```python
from build123d import *

# Parameters (mm, degrees)
SKETCH1_W               = 8
SKETCH1_H               = 4.5
SKETCH1_R               = 1.5
SKETCH1_W_2             = 65.532
SKETCH1_H_2             = 78.229021166
SKETCH1_R_2             = 1.599939077
SKETCH1_R_3             = 1.6
SKETCH1_R_4             = 1.599995589
SKETCH1_W_3             = 59.532
SKETCH1_H_3             = 64.229021166
BOSS_EXTRUDE1_DEPTH     = 3
SKETCH2_W               = 40
SKETCH2_H               = 4
BOSS_EXTRUDE2_DEPTH     = 30
CUT_EXTRUDE1_DEPTH      = 111.01120349
CUT_EXTRUDE1_DEPTH_BACK = 111.01120349
SKETCH3_R               = 2
FILLET2_R               = 17
FILLET3_R               = 12
SKETCH1_8_W             = 65.532
SKETCH1_8_H             = 78.229021166
SKETCH1_8_R             = 1.599939077
SKETCH1_8_R_2           = 1.6
SKETCH1_8_R_3           = 1.599995589
SKETCH1_8_W_2           = 59.532
SKETCH1_8_H_2           = 64.229021166
BOSS_EXTRUDE3_DEPTH     = 20
SKETCH5_R               = 2.5
CUT_EXTRUDE2_DEPTH      = 5
SKETCH7_W               = 58.229021166
SKETCH7_H               = 14
CUT_EXTRUDE3_DEPTH      = 111.01120349


with BuildPart() as part:
    # Sketch1 → Boss-Extrude1 (new body)
    # profile 1 of 11: a face of its own
    with BuildSketch(Plane(origin=(0, 0, 0), x_dir=(1, 0, 0), z_dir=(0, 1, 0))):
        with Locations((-4, 59.114510583)):
            Rectangle(SKETCH1_W, SKETCH1_H)
        with Locations(Location((-4, 59.114510583, 0), (0, 0, 270))):
            Circle(SKETCH1_R, mode=Mode.SUBTRACT)
    # profile 2 of 11: a face of its own
    with BuildSketch(Plane(origin=(0, 0, 0), x_dir=(1, 0, 0), z_dir=(0, 1, 0))):
        with Locations((4, 59.114510583)):
            Rectangle(SKETCH1_W, SKETCH1_H)
    # profile 3 of 11: a face of its own
    with BuildSketch(Plane(origin=(0, 0, 0), x_dir=(1, 0, 0), z_dir=(0, 1, 0))):
        Polygon((0, 56.864510583), (0, 39.114510583), (32.766, 39.114510583), (28.9648375, 56.864510583), (20.483, 56.864510583), (20.483, 61.364510583), (28.0011625, 61.364510583), (24.2, 79.114510583), (0, 79.114510583), (0, 61.364510583), (8, 61.364510583), (8, 56.864510583), align=None)
    # profile 4 of 11: a face of its own
    with BuildSketch(Plane(origin=(0, 0, 0), x_dir=(1, 0, 0), z_dir=(0, 1, 0))):
        Polygon((20.483, 56.864510583), (28.9648375, 56.864510583), (28.0011625, 61.364510583), (20.483, 61.364510583), align=None)
    # profile 5 of 11: a face of its own
    with BuildSketch(Plane(origin=(0, 0, 0), x_dir=(1, 0, 0), z_dir=(0, 1, 0))):
        Polygon((28.0011625, 61.364510583), (28.9648375, 56.864510583), (36.483, 56.864510583), (36.483, 61.364510583), align=None)
        with Locations(Location((32.483, 59.114510583, 0), (0, 0, 270))):
            Circle(SKETCH1_R, mode=Mode.SUBTRACT)
    # profile 6 of 11: a face of its own
    with BuildSketch(Plane(origin=(0, 0, 0), x_dir=(1, 0, 0), z_dir=(0, 1, 0))):
        with Locations((32.766, 0)):
            Rectangle(SKETCH1_W_2, SKETCH1_H_2)
        with Locations(Location((39.450944, -35.179510583, 0), (0, 0, 270))):
            Circle(SKETCH1_R_2, mode=Mode.SUBTRACT)
        with Locations(Location((20.574, -35.179510583, 0), (0, 0, 270))):
            Circle(SKETCH1_R_3, mode=Mode.SUBTRACT)
        with Locations(Location((39.37, 35.1758104, 0), (0, 0, 270))):
            Circle(SKETCH1_R_2, mode=Mode.SUBTRACT)
        with Locations(Location((20.574, 35.1758104, 0), (0, 0, 270))):
            Circle(SKETCH1_R_4, mode=Mode.SUBTRACT)
        with Locations((32.766, 0)):
            Rectangle(SKETCH1_W_3, SKETCH1_H_3, mode=Mode.SUBTRACT)
    # profile 7 of 11: a face of its own
    with BuildSketch(Plane(origin=(0, 0, 0), x_dir=(1, 0, 0), z_dir=(0, 1, 0))):
        Polygon((32.766, -39.114510583), (0, -39.114510583), (0, -56.864510583), (8, -56.864510583), (8, -61.364510583), (0, -61.364510583), (0, -79.114510583), (24.2, -79.114510583), (28.0011625, -61.364510583), (20.483, -61.364510583), (20.483, -56.864510583), (28.9648375, -56.864510583), align=None)
    # profile 8 of 11: a face of its own
    with BuildSketch(Plane(origin=(0, 0, 0), x_dir=(1, 0, 0), z_dir=(0, 1, 0))):
        Polygon((28.0011625, -61.364510583), (28.9648375, -56.864510583), (20.483, -56.864510583), (20.483, -61.364510583), align=None)
    # profile 9 of 11: a face of its own
    with BuildSketch(Plane(origin=(0, 0, 0), x_dir=(1, 0, 0), z_dir=(0, 1, 0))):
        Polygon((36.483, -56.864510583), (28.9648375, -56.864510583), (28.0011625, -61.364510583), (36.483, -61.364510583), align=None)
        with Locations(Location((32.483, -59.114510583, 0), (0, 0, 270))):
            Circle(SKETCH1_R, mode=Mode.SUBTRACT)
    # profile 10 of 11: a face of its own
    with BuildSketch(Plane(origin=(0, 0, 0), x_dir=(1, 0, 0), z_dir=(0, 1, 0))):
        with Locations((4, -59.114510583)):
            Rectangle(SKETCH1_W, SKETCH1_H)
    # profile 11 of 11: a face of its own
    with BuildSketch(Plane(origin=(0, 0, 0), x_dir=(1, 0, 0), z_dir=(0, 1, 0))):
        with Locations((-4, -59.114510583)):
            Rectangle(SKETCH1_W, SKETCH1_H)
        with Locations(Location((-4, -59.114510583, 0), (0, 0, 270))):
            Circle(SKETCH1_R, mode=Mode.SUBTRACT)
    extrude(amount=BOSS_EXTRUDE1_DEPTH)

    # Sketch2 → Boss-Extrude2 (add)
    with BuildSketch(Plane(origin=(0, 0, 0), x_dir=(1, 0, 0), z_dir=(0, 1, 0))):
        with Locations((4.2, -81.114510583)):
            Rectangle(SKETCH2_W, SKETCH2_H)
        with Locations((4.2, 81.114510583)):
            Rectangle(SKETCH2_W, SKETCH2_H)
    extrude(amount=BOSS_EXTRUDE2_DEPTH)

    # Sketch3 → Cut-Extrude1 (cut, two sides: drawn at the far end of the back side and taken through both)
    with BuildSketch(Plane.XY.offset(-CUT_EXTRUDE1_DEPTH_BACK)):
        with Locations((-7.8, 16)):
            Circle(SKETCH3_R)
        with BuildLine():
            Line((4.2, 18), (-7.8, 18))
            ThreePointArc((-7.8, 18), (-6.385786438, 17.414213562), (-5.8, 16))
            ThreePointArc((-5.8, 16), (-6.385786438, 14.585786438), (-7.8, 14))
            Line((-7.8, 14), (4.2, 14))
            ThreePointArc((4.2, 14), (2.2, 16), (4.2, 18))
        make_face()
        with Locations((4.2, 16)):
            Circle(SKETCH3_R)
        with Locations((14.2, 19.1)):
            Circle(SKETCH3_R)
    extrude(amount=CUT_EXTRUDE1_DEPTH + CUT_EXTRUDE1_DEPTH_BACK, mode=Mode.SUBTRACT)

    # Fillet2
    fillet2_edges = [part.edges().sort_by_distance(p)[0] for p in [
        (-15.8, 30, 81.114510583),
        (24.2, 30, 81.114510583),
        (24.2, 30, -81.114510583),
        (-15.8, 30, -81.114510583),
    ]]
    fillet(fillet2_edges, radius=FILLET2_R)

    # Fillet3
    fillet3_edges = [part.edges().sort_by_distance(p)[0] for p in [
        (-15.8, 0, 81.114510583),
        (-15.8, 0, -81.114510583),
    ]]
    fillet(fillet3_edges, radius=FILLET3_R)

    # Sketch1_8 → Boss-Extrude3 (add)
    with BuildSketch(Plane(origin=(0, 0, 0), x_dir=(1, 0, 0), z_dir=(0, 1, 0))):
        with Locations((32.766, 0)):
            Rectangle(SKETCH1_8_W, SKETCH1_8_H)
        with Locations(Location((39.450944, -35.179510583, 0), (0, 0, 270))):
            Circle(SKETCH1_8_R, mode=Mode.SUBTRACT)
        with Locations(Location((20.574, -35.179510583, 0), (0, 0, 270))):
            Circle(SKETCH1_8_R_2, mode=Mode.SUBTRACT)
        with Locations(Location((39.37, 35.1758104, 0), (0, 0, 270))):
            Circle(SKETCH1_8_R, mode=Mode.SUBTRACT)
        with Locations(Location((20.574, 35.1758104, 0), (0, 0, 270))):
            Circle(SKETCH1_8_R_3, mode=Mode.SUBTRACT)
        with Locations((32.766, 0)):
            Rectangle(SKETCH1_8_W_2, SKETCH1_8_H_2, mode=Mode.SUBTRACT)
    extrude(amount=BOSS_EXTRUDE3_DEPTH)

    # Sketch5 → Cut-Extrude2 (cut)
    with BuildSketch(Plane(origin=(0, 0, 0), x_dir=(1, 0, 0), z_dir=(0, 1, 0))):
        with Locations(Location((20.574, -35.179510583, 0), (0, 0, 270))):
            Circle(SKETCH5_R)
        with Locations(Location((39.450944, -35.179510583, 0), (0, 0, 270))):
            Circle(SKETCH5_R)
        with Locations(Location((20.574, 35.1758104, 0), (0, 0, 270))):
            Circle(SKETCH5_R)
        with Locations(Location((39.37, 35.1758104, 0), (0, 0, 270))):
            Circle(SKETCH5_R)
    extrude(amount=CUT_EXTRUDE2_DEPTH, mode=Mode.SUBTRACT)

    # Sketch7 → Cut-Extrude3 (cut, through all)
    with BuildSketch(Plane(origin=(0, 0, 0), x_dir=(0, 0, -1), z_dir=(1, 0, 0))):
        with Locations((0, 10)):
            Rectangle(SKETCH7_W, SKETCH7_H)
    extrude(amount=CUT_EXTRUDE3_DEPTH, mode=Mode.SUBTRACT)


solid = part.part
```
Input: part model. Units: mm. Frame: model coordinates. A direction names the side the tool comes from. Give positions to 0.01 mm unless a question says otherwise; leave off trailing zeros. Write each loop counter-clockwise with the first axis right and the second up, starting at its lowest first coordinate (ties: lowest second). Pieces come first, ordered by that corner, then holes. Notation, with made-up numbers: (-9, -14.5) - (47, -14.5) arc R19 ccw to (47, 0.5) - close; hole circle Ø6 at (37.25, 4.25). An arc over 180 degrees is marked (long way). Write item = value, one per line. Start each with the question number.
1) Reachability of faces 1 (the face through (38.8, 5, -33.5)), 2 (the face through (-9.8, 16, -81.1)), 3 (the face through (3, 2.5, 0.1)), 4 (the face through (24.2, 6, 81)), 5 (the face through (-2, 18, 81)) from +Z, -Z, +X, -X, +Y, -Y: full face, straight path, thin tool, end or side. Return the list, or none.
2) Cut plane A-A (y = 10.5). Return loops of the section in (x, z), and give its area (3 significant figures).
3) Pin query (flat end, axial travel): pin 1 (6 mm diameter, centred on x = 30, y = 12.5, fed in from +Z); pin 2 (3.5 mm diameter, centred on x = 32, y = 1, fed in from -Z); pin 3 (3.5 mm diameter, centred on x = -4, z = 59.11, fed in from +Y); pin 4 (3 mm diameter, centred on x = 20.57, z = 35.18, fed in from -Y). Return the tip coordinate at first contact, or that it passes through.
4) Draft query along X for faces 6 (the face through (64, 10, 29.115)), 7 (the face through (19.05, 2.46, -37.16)), 8 (the face through (30.89, 1.48, -47.87)), 9 (the face through (-10.95, 24.89, -81.14)). Return one class per face: pulls with the +X half, pulls with the -X half, needs draft (parallel to the pull), parting line crosses it, or undercut.
5) Cut plane B-B (z = -17.5). Return loops of the section in (x, y), and give its area (3 significant figures).
6) Cut plane D-D (y = 25.5). Return loops of the section in (x, z), and give its area (3 significant figures).
7) Material intervals for L1, parallel to Z at x = 17.5, y = 16.5; L2, parallel to Z at x = 36, y = 10.5; L3, parallel to Z at x = -6, y = 11.5, sorted ascending. Write a range as [from, to].
8) Cut plane C-C (x = 14.2). Return loops of the section in (y, z).
Answers follow:
q1.face_1 = -Y
q1.face_2 = +Z, -Z
q1.face_3 = +Y, -Y
q1.face_4 = +Z, +X, +Y, -Y
q1.face_5 = +Z
q2.outline = (-15.71, -83.11) - (24.2, -83.11) - (24.2, -79.11) - (-15.71, -79.11) - close; (-15.71, 79.11) - (24.2, 79.11) - (24.2, 83.11) - (-15.71, 83.11) - close; (0, -39.11) - (65.53, -39.11) - (65.53, -29.11) - (62.53, -29.11) - (62.53, -32.11) - (3, -32.11) - (3, -29.11) - (0, -29.11) - close; (0, 29.11) - (3, 29.11) - (3, 32.11) - (62.53, 32.11) - (62.53, 29.11) - (65.53, 29.11) - (65.53, 39.11) - (0, 39.11) - close; hole circle Ø3.2 at (20.57, -35.18); hole circle Ø3.2 at (20.57, 35.18); hole circle Ø3.2 at (39.37, -35.18); hole circle Ø3.2 at (39.45, 35.18)
q2.area = 1,240 mm^2
q3.pin_1 = 39.11
q3.pin_2 = -61.36
q3.pin_3 = 3
q3.pin_4 = through
q4.face_6 = needs draft
q4.face_7 = undercut
q4.face_8 = pulls with the +X half
q4.face_9 = pulls with the -X half
q5.outline = (0, 0) - (3, 0) - (3, 3) - (0, 3) - close; (0, 17) - (3, 17) - (3, 20) - (0, 20) - close; (62.53, 0) - (65.53, 0) - (65.53, 3) - (62.53, 3) - close; (62.53, 17) - (65.53, 17) - (65.53, 20) - (62.53, 20) - close
q5.area = 36.0 mm^2
q6.outline = (-10.32, -83.11) - (18.72, -83.11) - (18.72, -79.11) - (-10.32, -79.11) - close; (-10.32, 79.11) - (18.72, 79.11) - (18.72, 83.11) - (-10.32, 83.11) - close
q6.area = 232 mm^2
q7.L1 = [-83.11, -79.11], [-39.11, -32.11], [32.11, 39.11], [79.11, 83.11]
q7.L2 = [-39.11, -32.11], [32.11, 39.11]
q7.L3 = [-83.11, -79.11], [79.11, 83.11]
q8.outline = (0, -83.11) - (17.1, -83.11) - (17.1, -79.11) - (3, -79.11) - (3, -39.11) - (20, -39.11) - (20, -32.11) - (0, -32.11) - close; (0, 32.11) - (20, 32.11) - (20, 39.11) - (3, 39.11) - (3, 79.11) - (17.1, 79.11) - (17.1, 83.11) - (0, 83.11) - close; (21.1, -83.11) - (28.49, -83.11) - (28.49, -79.11) - (21.1, -79.11) - close; (21.1, 79.11) - (28.49, 79.11) - (28.49, 83.11) - (21.1, 83.11) - close
